CAD build for the part. Positions are in the model's coordinates, mm. Coordinates: 2 decimals unless noted, no trailing zeros. Loops run counter-clockwise (first coordinate to the right, second up) from the corner with the lowest first, then second, coordinate; pieces in that order, holes last. Notation, with made-up numbers: (-34, 18.5) -> (7, 18.5) arc R27 ccw to (7, 46.5) -> close; hole circle Ø6 at (1, -17). An arc over 180 degrees is marked (long way). Answer as CSV lines item,"result". Start each with the question number.
```python
from build123d import *
from build123d.topology import SkipClean

# Parameters (mm, degrees)
SKETCH1_R           = 2
BOSS_EXTRUDE1_DEPTH = 42
BOSS_EXTRUDE2_DEPTH = 10
CUT_EXTRUDE1_DEPTH  = 7
BOSS_EXTRUDE4_DEPTH = 3
SKETCH5_R           = 1.5
CUT_EXTRUDE3_DEPTH  = 54.708670792
SKETCH6_W           = 11.822480184
SKETCH6_H           = 12.15707868
CUT_EXTRUDE5_DEPTH  = 54.708670792
FILLET4_R           = 1
FILLET5_R           = 1
SKETCH7_W           = 34.513514199
SKETCH7_H           = 14.72292105
CUT_EXTRUDE6_DEPTH  = 50.84257119
SKETCH8_W           = 4
SKETCH8_H           = 12.808527321
SKETCH8_R           = 1.5
BOSS_EXTRUDE5_DEPTH = 3
FILLET6_R           = 1


with BuildPart() as part:
    # Sketch1 → Boss-Extrude1 (new body)
    with BuildSketch(Plane(origin=(0, 0, 0), x_dir=(0, 0, -1), z_dir=(1, 0, 0))):
        with Locations(Location((-12.6584653, 7.000514901, 0), (0, 0, 180))):
            Circle(SKETCH1_R)
    extrude(amount=BOSS_EXTRUDE1_DEPTH)

    # Sketch2 → Boss-Extrude2 (add)
    with BuildSketch(Plane.ZY):
        with BuildLine():
            Line((10.6584653, 7.000514901), (10.6584653, 13.760469307))
            ThreePointArc((10.6584653, 13.760469307), (12.6584653, 15.760469307), (14.6584653, 13.760469307))
            Line((14.6584653, 13.760469307), (14.6584653, 7.000514901))
            ThreePointArc((14.6584653, 7.000514901), (12.6584653, 5.000514901), (10.6584653, 7.000514901))
        make_face()
    extrude(amount=-BOSS_EXTRUDE2_DEPTH)

    # Sketch3 → Cut-Extrude1 (cut)
    with SkipClean():  # the faces are left unmerged after this step: merging them gives an invalid solid
        with BuildSketch(Plane.ZY):
            with BuildLine():
                Line((10.6584653, 7.000514901), (10.6584653, 13.760469307))
                ThreePointArc((10.6584653, 13.760469307), (12.6584653, 15.760469307), (14.6584653, 13.760469307))
                Line((14.6584653, 13.760469307), (14.6584653, 7.000514901))
                ThreePointArc((14.6584653, 7.000514901), (12.6584653, 9.000514901), (10.6584653, 7.000514901))
            make_face()
        extrude(amount=-CUT_EXTRUDE1_DEPTH, mode=Mode.SUBTRACT)

    # Sketch4 → Boss-Extrude4 (add)
    with SkipClean():  # the faces are left unmerged after this step: merging them gives an invalid solid
        with BuildSketch(Plane.ZY.offset(-7)):
            with BuildLine():
                Line((10.6584653, 36.009876522), (10.6584653, 13.760469307))
                ThreePointArc((10.6584653, 13.760469307), (12.6584653, 15.760469307), (14.6584653, 13.760469307))
                Line((14.6584653, 13.760469307), (14.6584653, 36.009876522))
                Line((14.6584653, 36.009876522), (10.6584653, 36.009876522))
            make_face()
            with BuildLine():
                ThreePointArc((10.6584653, 36.009876522), (12.6584653, 38.009876522), (14.6584653, 36.009876522))
                Line((14.6584653, 36.009876522), (10.6584653, 36.009876522))
            make_face()
        extrude(amount=-BOSS_EXTRUDE4_DEPTH)

    # Sketch5 → Cut-Extrude3 (cut, through all)
    with SkipClean():  # the faces are left unmerged after this step: merging them gives an invalid solid
        with BuildSketch(Plane.ZY.offset(-7)):
            with Locations((12.706639089, 22.91954594)):
                Circle(SKETCH5_R)
        extrude(amount=-CUT_EXTRUDE3_DEPTH, mode=Mode.SUBTRACT)

    # Sketch6 → Cut-Extrude5 (cut, through all)
    with SkipClean():  # the faces are left unmerged after this step: merging them gives an invalid solid
        with BuildSketch(Plane.ZY.offset(-7)):
            with Locations((12.630555797, 32.616849438)):
                Rectangle(SKETCH6_W, SKETCH6_H)
        extrude(amount=-CUT_EXTRUDE5_DEPTH, mode=Mode.SUBTRACT)

    # Fillet4
    fillet4_edges = [part.edges().sort_by_distance(p)[0] for p in [
        (8.5, 26.538310098, 14.6584653),
    ]]
    fillet(fillet4_edges, radius=FILLET4_R)

    # Fillet5
    fillet5_edges = [part.edges().sort_by_distance(p)[0] for p in [
        (8.5, 26.538310098, 10.6584653),
    ]]
    fillet(fillet5_edges, radius=FILLET5_R)

    # Sketch7 → Cut-Extrude6 (cut, through all)
    with BuildSketch(Plane(origin=(0, 0, 10.6584653), x_dir=(-1, 0, 0), z_dir=(0, 0, -1))):
        with Locations((-29.975495684, 6.364049631)):
            Rectangle(SKETCH7_W, SKETCH7_H)
    extrude(amount=-CUT_EXTRUDE6_DEPTH, mode=Mode.SUBTRACT)

    # Sketch8 → Boss-Extrude5 (add)
    with SkipClean():  # the faces are left unmerged after this step: merging them gives an invalid solid
        with BuildSketch(Plane.ZY.offset(-7)):
            with Locations((12.6584653, 25.427627083)):
                Rectangle(SKETCH8_W, SKETCH8_H)
            with Locations((12.6584653, 28.953962247)):
                Circle(SKETCH8_R, mode=Mode.SUBTRACT)
        extrude(amount=-BOSS_EXTRUDE5_DEPTH)

    # Fillet6
    fillet6_edges = [part.edges().sort_by_distance(p)[0] for p in [
        (8.5, 31.831890743, 14.6584653),
        (8.5, 31.831890743, 10.6584653),
    ]]
    fillet(fillet6_edges, radius=FILLET6_R)


solid = part.part
```
Q1. Pin check, flat tips, straight feed: pin 1 Ø1 at (x, y) = (6, 12) entering from +Z; pin 2 Ø1.2 at (y, z) = (23, 12) entering from +X. Stop position of each tip, or through.
Q2. Saw through at A-A (y = 27.75). List the corners of the cut face in (x, z).
Q3. Probe probe 1 along X at (y, z) = (13.75, 12.9); probe 2 along Y at (x, z) = (9, 12.45); probe 3 along Y at (x, z) = (8.5, 13.45). List the from-to ranges inside material, lowest first. Write a range as from..to.
Q4. Saw through at D-D (y = 10.5). List the corners of the cut face in (x, z), and give its area (3 significant figures).
Q5. Saw through at C-C (x = 8.5). List the corners of the cut face in (y, z).
Q6. Two-plate mould, pull along Z, no slides. Class faces 1 (the flat face through (10, 20, 13)), 2 (the cylindrical face through (8.48, 30.44, 12.46)), 3 (the flat face through (8, 19, 14.658)): pulls with the +Z half, pulls with the -Z half, needs draft (parallel to the pull), parting line crosses it, or undercut.
Q7. Saw through at B-B (z = 12.1). List the corners of the cut face in (x, y).
Ans:
1,pin 1,"passes through"
1,pin 2,"stops at x = 10"
2,outline,"(7, 10.66) -> (10, 10.66) -> (10, 11.76) -> (7, 11.76) -> close; (7, 13.55) -> (10, 13.55) -> (10, 14.66) -> (7, 14.66) -> close"
3,probe 1,"x = 7..10"
3,probe 2,"y = 5.01..27.47, 30.44..31.83"
3,probe 3,"y = 5.16..27.68, 30.23..31.83"
4,outline,"(7, 10.66) -> (10, 10.66) -> (10, 14.66) -> (7, 14.66) -> close"
4,area,"12.0 mm²"
5,outline,"(7, 10.66) -> (30.83, 10.66) arc R1 ccw to (31.83, 11.66) -> (31.83, 13.66) arc R1 ccw to (30.83, 14.66) -> (7, 14.66) arc R2 ccw to start; hole circle Ø3 at (28.95, 12.66)"
6,face 1,"needs draft"
6,face 2,"undercut"
6,face 3,"pulls with the +Z half"
7,outline,"(0, 5.08) -> (12.72, 5.08) -> (12.72, 8.92) -> (10, 8.92) -> (10, 27.56) -> (7, 27.56) -> (7, 8.92) -> (0, 8.92) -> close; (7, 30.35) -> (10, 30.35) -> (10, 31.83) -> (7, 31.83) -> close"
